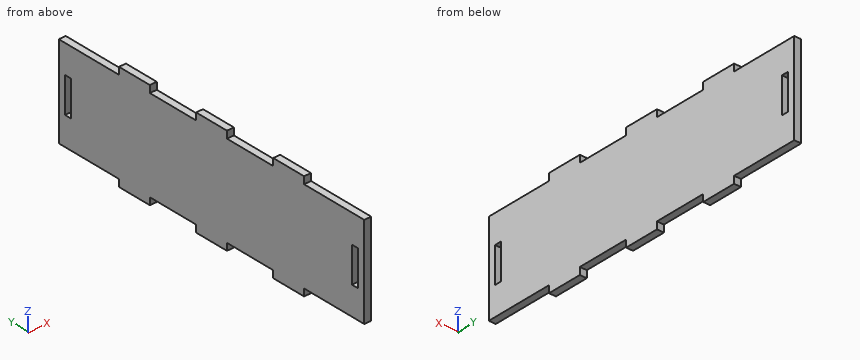
Solid Edge part; units mm, degrees
sketch "Sketch1" plane through (0, 0, 0) normal (1, 0, 0) x (0, 1, 0)
  line L0 (64.5, -13) -> (45, -13)
  line L1 (45, -13) -> (45, -15)
  line L2 (45, -15) -> (35, -15)
  line L3 (35, -15) -> (35, -13)
  line L4 (35, -13) -> (20, -13)
  line L5 (20, -13) -> (20, -15)
  line L6 (20, -15) -> (10, -15)
  line L7 (10, -15) -> (10, -13)
  line L8 (10, -13) -> (-5, -13)
  line L9 (-5, -13) -> (-5, -15)
  line L10 (-5, -15) -> (-15, -15)
  line L11 (-15, -15) -> (-15, -13)
  line L12 (-15, -13) -> (-34.5, -13)
  line L13 (-34.5, -13) -> (-34.5, 13)
  line L14 (-34.5, 13) -> (-15, 13)
  line L15 (-15, 13) -> (-15, 15)
  line L16 (-15, 15) -> (-5, 15)
  line L17 (-5, 15) -> (-5, 13)
  line L18 (-5, 13) -> (10, 13)
  line L19 (10, 13) -> (10, 15)
  line L20 (10, 15) -> (20, 15)
  line L21 (20, 15) -> (20, 13)
  line L22 (20, 13) -> (35, 13)
  line L23 (35, 13) -> (35, 15)
  line L24 (35, 15) -> (45, 15)
  line L25 (45, 15) -> (45, 13)
  line L26 (45, 13) -> (64.5, 13)
  line L27 (64.5, 13) -> (64.5, -13)
  line L28 (-32.5, -5) -> (-30.5, -5)
  line L29 (-32.5, 5) -> (-32.5, -5)
  line L30 (-30.5, 5) -> (-32.5, 5)
  line L31 (-30.5, -5) -> (-30.5, 5)
  line L32 (62.5, -5) -> (62.5, 5)
  line L33 (60.5, -5) -> (62.5, -5)
  line L34 (60.5, 5) -> (60.5, -5)
  line L35 (62.5, 5) -> (60.5, 5)
extrude "ExtrudedProtrusion_1" add sketch "Sketch1" along normal blind 2
properties material "Acrylic, high impact grade"
For this review, take the finished solid that the model builds, in its own axes (mm). Give positions to 0.01 mm unless a question says otherwise; leave off trailing zeros. Write each loop counter-clockwise with the first axis right and the second up, starting at its lowest first coordinate (ties: lowest second). Pieces come first, ordered by that corner, then holes. Notation, with made-up numbers: M 16.5,44 L 68.5,44 A9 cw 68.5,48 Z; hole C 87,13.5 d5. An arc over 180 degrees is marked long. Answer as a JSON object with one key per item and string values. Group by question number.
Item 1: Consider section A-A on z = 3.75. Write out the cut boundary in (x, y).
Item 2: Consider section C-C on y = -24.5. Write out the cut boundary in (x, z), plus the area to 3 significant figures.
Item 3: For pin 1 Ø0.6 at (x, z) = (1, 13.5) entering from +Y; pin 2 Ø1 at (x, z) = (1, -14.5) entering from -Y; pin 3 Ø0.6 at (x, y) = (1, 58) entering from +Z, all flat-tipped, find the tip position at first contact; note any pin that passes through.
Item 4: For probe 1 along Y at (x, z) = (1.25, -0.75); probe 2 along Z at (x, y) = (1.1, 22), list the stretches that pass through material, from the lowest coordinate up. Write a range as [from, to].
Item 5: Consider section B-B on x = 1. Count the separate pieces of the cut face and the enclosed holes in it, plus the area to 3 significant figures.
Check result:
{
 "1": {"outline": "M 0,-34.5 L 2,-34.5 L 2,-32.5 L 0,-32.5 Z; M 0,-30.5 L 2,-30.5 L 2,60.5 L 0,60.5 Z; M 0,62.5 L 2,62.5 L 2,64.5 L 0,64.5 Z"},
 "2": {"outline": "M 0,-13 L 2,-13 L 2,13 L 0,13 Z", "area": "52.0 mm^2"},
 "3": {"pin 1": "stops at y = 45", "pin 2": "stops at y = -15", "pin 3": "stops at z = 13"},
 "4": {"probe 1": "y = [-34.5, -32.5], [-30.5, 60.5], [62.5, 64.5]", "probe 2": "z = [-13, 13]"},
 "5": {"separate pieces": "1", "enclosed holes": "2", "area": "2,650 mm^2"}
}
